Geometry check sheet. Reference: the model listing, model coordinates, mm. Coordinates: 2 decimals unless noted, no trailing zeros. Order: outer loops, then holes, each group sorted by start corner. A loop starts at its lowest first (then second) coordinate and runs counter-clockwise, first axis right, second up. Notation, with made-up numbers: (76.5, 48) - (107.5, 48) arc R21 ccw to (107.5, 60) - close; hole circle Ø11 at (81, -39). An arc over 180 degrees is marked (long way). Use CSV: the item, a comma, the result in double quotes. Start each with the question number.
1) Thickness scan on probe 1 along Y at (x, z) = (-27.5, 6); probe 2 along X at (y, z) = (10, 49); probe 3 along X at (y, z) = (6.5, 48.5). Record the ranges inside material, lowest first. Write a range as [from, to].
2) Sectioned sample at D-D, the plane y = 24. Record the cut outline in (x, z), and give its area (3 significant figures).
3) Sectioned sample at B-B, the plane y = 16.5. Record the cut outline in (x, z).
4) Sectioned sample at C-C, the plane x = -8. Record the cut outline in (y, z).
from build123d import *

# Parameters (mm, degrees)
F1_DEPTH = 25.4
F3_DEPTH = 25.4
F4_DEPTH = 25.4
F5_DEPTH = 47.752


with BuildPart() as f1:
    # F0 (on Front) → F1 (new body)
    with BuildSketch(Plane.XZ):
        Polygon((-57.9928606749, 0), (0, 0), (-29.787896201, 55.1148019731), align=None)
    extrude(amount=F1_DEPTH)

    # F2 (on face) → F3 (join)
    with BuildSketch(Plane.XZ):
        with BuildLine():
            ThreePointArc((-32.3781482875, 55.6904152036), (-40.4396180835, 25.7523156056), (-57.7050559223, 0))
            ThreePointArc((-57.7050559223, 0), (-28.8525279611, 4.8719261638), (0, 0))
            ThreePointArc((0, 0), (-20.8306687823, 25.146606075), (-32.3781482875, 55.6904152036))
        make_face()
    extrude(amount=-F3_DEPTH)

    # F4 (cut): faces of the model
    f4_faces = [f1.faces().sort_by_distance(p)[0] for p in [
        (-44.4714868788, 0, 22.9050360722),
        (-28.8525279611, 0, 1.9534765457),
        (-18.405809999, 0, 28.5034341287),
        (-44.4714868788, 0, 22.9050360722),
        (-28.8525279611, 0, 1.9534765457),
        (-18.405809999, 0, 28.5034341287),
        (-28.8525279611, 0, 1.9534765457),
    ]]
    extrude(f4_faces, amount=-F4_DEPTH, mode=Mode.SUBTRACT)

    # F5 (cut): a face of the model
    f5_faces = [f1.faces().sort_by_distance(p)[0] for p in [
        (-30.2908637414, -25.4, 17.8560870297),
    ]]
    extrude(f5_faces, amount=-F5_DEPTH, mode=Mode.SUBTRACT)


solid = f1.part
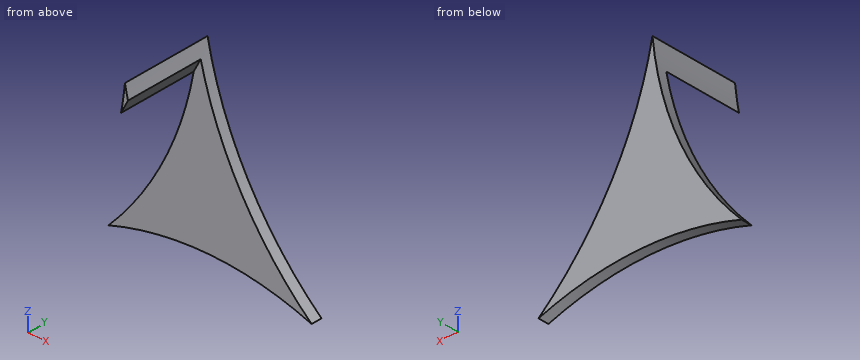
Evaluation:
1,probe 1,"[22.35, 25.4]"
1,probe 2,"[-33.29, -32.92]"
1,probe 3,"[-33.37, -33.17]"
2,outline,"(-57.71, 0) arc R87.87 cw to (0, 0) arc R99.3 cw to (-32.38, 55.69) arc R95.07 cw to start"
2,area,"979 mm²"
3,outline,"(-33.48, 47.9) - (-31.51, 51.75) arc R99.3 cw to (-32.38, 55.69) arc R95.07 cw to start"
4,outline,"(22.35, 2.36) - (25.4, 2.36) - (25.4, 7.76) - (22.35, 7.76) - close"
